from build123d import *

# Parameters (mm, degrees)
BOSS_EXTRU_1_DEPTH      = 12.15
ESQUISSE2_R             = 1
ENL_V_MAT_EXTRU_1_DEPTH = 28.596900188
ESQUISSE4_R             = 0.5
BOSS_EXTRU_4_DEPTH      = 4
ESQUISSE5_R             = 2.475
ESQUISSE5_R_2           = 0.75
BOSS_EXTRU_5_DEPTH      = 3
CONG_1_R                = 0.5


with BuildPart() as part:
    # Esquisse1 → Boss.-Extru.1 (new body)
    with BuildSketch(Plane.XY):
        Polygon((11.5, -17.2), (-11.5, -17.2), (-11.5, 0), (-16, 0), (-16, 1.72), (-11.5, 1.72), (-11.5, 4.22), (-10.567959043, 4.582352941), (-9.297370807, 7.3), (11.5, 7.3), (11.5, 1.72), (16, 1.72), (16, 0), (11.5, 0), align=None)
    extrude(amount=BOSS_EXTRU_1_DEPTH)

    # Esquisse2 → Enlèv. mat.-Extru.1 (cut, through all)
    with BuildSketch(Plane(origin=(0, 1.72, 0), x_dir=(1, 0, 0), z_dir=(0, 1, 0))):
        with Locations(Location((-14, -6.075, 0), (0, 0, 180))):
            Circle(ESQUISSE2_R)
        with Locations(Location((14, -6.075, 0), (0, 0, 180))):
            Circle(ESQUISSE2_R)
    extrude(amount=-ENL_V_MAT_EXTRU_1_DEPTH, mode=Mode.SUBTRACT)

    # Esquisse4 → Boss.-Extru.4 (add)
    with BuildSketch(Plane(origin=(11.5, 0, 0), x_dir=(0, 0, -1), z_dir=(1, 0, 0))):
        with Locations((-6.075, -14.6)):
            Circle(ESQUISSE4_R)
        with Locations((-7.025, -14.6)):
            Circle(ESQUISSE4_R)
        with Locations((-5.125, -14.6)):
            Circle(ESQUISSE4_R)
    extrude(amount=BOSS_EXTRU_4_DEPTH)

    # Esquisse5 → Boss.-Extru.5 (add)
    with BuildSketch(Plane(origin=(0, 7.3, 0), x_dir=(1, 0, 0), z_dir=(0, 1, 0))):
        with Locations((6.5, -6.075)):
            Circle(ESQUISSE5_R)
        with Locations(Location((6.5, -6.075, 0), (0, 0, 180))):
            Circle(ESQUISSE5_R_2, mode=Mode.SUBTRACT)
    extrude(amount=BOSS_EXTRU_5_DEPTH)

    # Congé1
    cong_1_edges = [part.edges().sort_by_distance(p)[0] for p in [
        (16, 0.86, 12.15),
        (0, -17.2, 0),
        (-11.5, -8.6, 0),
        (13.75, 1.72, 12.15),
        (-13.75, 0, 0),
        (-16, 0.86, 0),
        (-13.75, 1.72, 0),
        (-11.5, 2.97, 0),
        (-11.033979521, 4.401176471, 0),
        (-9.932664925, 5.941176471, 0),
        (1.101314596, 7.3, 0),
        (11.5, 4.51, 12.15),
        (11.5, 4.51, 0),
        (13.75, 1.72, 0),
        (16, 0.86, 0),
        (13.75, 0, 0),
        (11.5, -8.6, 0),
        (1.101314596, 7.3, 12.15),
        (-9.932664925, 5.941176471, 12.15),
        (11.5, -17.2, 6.075),
        (-11.5, -17.2, 6.075),
        (-11.5, 0, 6.075),
        (-11.5, 1.72, 6.075),
        (-11.5, 4.22, 6.075),
        (-10.567959043, 4.582352941, 6.075),
        (-9.297370807, 7.3, 6.075),
        (11.5, 7.3, 6.075),
        (11.5, 1.72, 6.075),
        (11.5, 0, 6.075),
        (-11.033979521, 4.401176471, 12.15),
        (-11.5, 2.97, 12.15),
        (-13.75, 1.72, 12.15),
        (-16, 0.86, 12.15),
        (-13.75, 0, 12.15),
        (11.5, -8.6, 12.15),
        (-11.5, -8.6, 12.15),
        (0, -17.2, 12.15),
        (13.75, 0, 12.15),
    ]]
    fillet(cong_1_edges, radius=CONG_1_R)


solid = part.part
Design review of the part built by this model. Coordinates are the model's own, in mm. A direction names the side the tool comes from. Round coordinates to 2 decimals unless told otherwise and drop trailing zeros. Loops run counter-clockwise (first coordinate to the right, second up) from the corner with the lowest first, then second, coordinate; pieces in that order, holes last. Notation, with made-up numbers: (37, -32.5) - (90, -32.5) arc R31 cw to (90, -7.5) - close; hole circle Ø8 at (88, 49). An arc over 180 degrees is marked (long way). One line per item, written item: value. Start each with the question number.
1) Insertion check: pin 1 Ø0.5 at (y, z) = (3, 3.5) entering from -X; pin 2 Ø2 at (x, z) = (-8, 10) entering from +Y; pin 3 Ø0.5 at (y, z) = (-14.5, 5.5) entering from +X. Each pin has a flat end and moves straight along its axis. Give the tip position at first contact, or say it passes through.
2) To check wall thickness, follow L1, parallel to Z at x = 14, y = 0.6 (3 decimals); L2, parallel to Z at x = 6.5, y = 8.9 (3 decimals); L3, parallel to Y at x = -6, z = 10.5. State the ranges of each line that lie inside material, in increasing order. Write a range as from..to.
3) Consider section D-D on z = 2.5. Give the boundary of the cut face in (x, y), then the cut area to 3 significant figures.
4) Consider section C-C on x = 14. Give the boundary of the cut face in (y, z) (3 decimals).
5) For faces 4 (the cylindrical face through (7.095, 8.779, 5.619)), 5 (the flat face through (-11.5, -9, 6)), 6 (the flat face through (14, 0, 4.8)), list the 3-axis set-ups (+Z, -Z, +X, -X, +Y, -Y) from which the entire face can be reached by the end or side of a thin tool; tool diameter is ignored.
6) Draft analysis for pull direction Z (two halves, no side actions). For faces 1 (the cylindrical face through (8.786, 8.779, 7.023)), 2 (the cylindrical face through (-14.924, 0.872, 5.692)), 3 (the cylindrical face through (-9.81, 5.84, 12.01)), state which applies: +Z half, -Z half, draft (parallel to the pull), parting line (faces both ways), or undercut.
7) Consider section A-A on x = -14. Give the boundary of the cut face in (y, z) (3 decimals).
8) Consider section B-B on y = -12.25. Give the boundary of the cut face in (x, z).
Reported:
1. pin 1: stops at x = -11.5
1. pin 2: stops at y = 7.3
1. pin 3: stops at x = 15.5
2. L1: z = 0..5.075, 7.075..12.15
2. L2: z = 3.6..5.325, 6.825..8.55
2. L3: y = -17.2..7.3
3. outline: (-16, 0) - (-12, 0) arc R0.5 cw to (-11.5, -0.5) - (-11.5, -16.7) arc R0.5 ccw to (-11, -17.2) - (11, -17.2) arc R0.5 ccw to (11.5, -16.7) - (11.5, -0.5) arc R0.5 cw to (12, 0) - (16, 0) - (16, 1.72) - (12, 1.72) arc R0.5 cw to (11.5, 2.22) - (11.5, 6.8) arc R0.5 ccw to (11, 7.3) - (-8.98, 7.3) arc R0.5 ccw to (-9.43, 7.01) - (-10.48, 4.76) arc R0.5 cw to (-10.75, 4.51) - (-11.18, 4.34) arc R0.5 ccw to (-11.5, 3.88) - (-11.5, 2.22) arc R0.5 cw to (-12, 1.72) - (-16, 1.72) - close
3. area: 575 mm^2
4. outline: (-14.756, 5.6) arc R0.5 ccw (long way) to (-14.444, 5.6) arc R0.5 ccw to (-14.444, 6.55) arc R0.5 ccw (long way) to (-14.756, 6.55) arc R0.5 ccw to start; (0, 0.5) arc R0.5 ccw to (0.5, 0) - (1.22, 0) arc R0.5 ccw to (1.72, 0.5) - (1.72, 5.075) - (0, 5.075) - close; (0, 7.075) - (1.72, 7.075) - (1.72, 11.65) arc R0.5 ccw to (1.22, 12.15) - (0.5, 12.15) arc R0.5 ccw to (0, 11.65) - close
5. face 4: +Y
5. face 5: +Z, -Z, -X, -Y
5. face 6: +Z, -Z, +X
6. face 1: parting line
6. face 2: undercut
6. face 3: +Z half
7. outline: (0, 0.5) arc R0.5 ccw to (0.5, 0) - (1.22, 0) arc R0.5 ccw to (1.72, 0.5) - (1.72, 5.075) - (0, 5.075) - close; (0, 7.075) - (1.72, 7.075) - (1.72, 11.65) arc R0.5 ccw to (1.22, 12.15) - (0.5, 12.15) arc R0.5 ccw to (0, 11.65) - close
8. outline: (-11.5, 0.5) arc R0.5 ccw to (-11, 0) - (11, 0) arc R0.5 ccw to (11.5, 0.5) - (11.5, 11.65) arc R0.5 ccw to (11, 12.15) - (-11, 12.15) arc R0.5 ccw to (-11.5, 11.65) - close
